Check sheet for the modelled part. Datum: model origin and axes. Units: mm. Face numbers are marked on the shaded views. Give positions to 0.01 mm unless a question says otherwise; leave off trailing zeros. Write each loop counter-clockwise with the first axis right and the second up, starting at its lowest first coordinate (ties: lowest second). Pieces come first, ordered by that corner, then holes. Notation, with made-up numbers: (51.5, 33) -> (62.5, 33) arc R21 ccw to (62.5, 39) -> close; hole circle Ø6 at (34.25, 73). An arc over 180 degrees is marked (long way). Use a Markdown table: item, result. Add a question column.
1. Cross-section at B-B (x = 0). Enter the section's corners in (y, z).
2. Cross-section at A-A (y = 0). Enter the section's corners in (x, z).
3. Scan lines: probe 1 along Y at (x, z) = (0, 12.5); probe 2 along Z at (x, y) = (7, 16.5); probe 3 along X at (y, z) = (-14, 8.25). Record each from-to range of solid material in increasing order. Write a range as [from, to].
4. Release check for a two-part mould opening along X. For the marked faces 1, 2 and 3 record: released by +X, released by -X, zero draft, split by the parting line, or undercut.
5. Cross-section at C-C (z = 9). Enter the section's corners in (x, y), then the cut area to 3 significant figures.
6. Gauge pin test, flat ends, axial feed: P1, Ø1.1, axis at x = -28, z = 15, coming from the -Y side; P2, Ø10, axis at x = -13.5, z = 7, coming from the +Y side; P3, Ø1.6, axis at x = 19.5, z = 19, coming from the -Y side; P4, Ø6, axis at x = -10.5, z = 3, coming from the -Y side. Record the tip position at first contact, or that the pin passes through.
from build123d import *

# Parameters (mm, degrees)
F0_R      = 29
F4_DEPTH  = 20
F5_SIZE   = 1
F1_R      = 28
F6_DEPTH  = 18
F2_W      = 5
F2_H      = 14
F7_DEPTH  = 20.1
F3_W      = 10.5
F3_H      = 2.55
F8_DEPTH  = 42.4
F9_W      = 46.34465
F9_H      = 65.188974
F10_DEPTH = 7
F11_W     = 30
F11_H     = 4
F12_DEPTH = 45


with BuildPart() as f4:
    # F0 (on Top) → F4 (new body)
    with BuildSketch(Plane.XY):
        Circle(F0_R)
    extrude(amount=F4_DEPTH)

    # F5
    f5_edges = [f4.edges().sort_by_distance(p)[0] for p in [
        (-29, 0, 20),
    ]]
    chamfer(f5_edges, length=F5_SIZE)

    # F1 (on Top) → F6 (cut)
    with BuildSketch(Plane.XY):
        Circle(F1_R)
    extrude(amount=F6_DEPTH, mode=Mode.SUBTRACT)

    # F2 (on face) → F7 (cut)
    with BuildSketch(Plane.XY):
        with Locations((18.5, 8.5)):
            Rectangle(F2_W, F2_H)
        with Locations((18.5, -8.5)):
            Rectangle(F2_W, F2_H)
    extrude(amount=F7_DEPTH, mode=Mode.SUBTRACT)

    # F3 (on Right) → F8 (cut)
    with BuildSketch(Plane.YZ):
        with Locations((-11.250031, 14.775)):
            Rectangle(F3_W, F3_H)
    extrude(amount=-F8_DEPTH, mode=Mode.SUBTRACT)

    # F9 (on Top) → F10 (cut)
    with BuildSketch(Plane.XY):
        Rectangle(F9_W, F9_H)
    extrude(amount=F10_DEPTH, mode=Mode.SUBTRACT)

    # F11 (on Right) → F12 (cut, symmetric)
    with BuildSketch(Plane.YZ):
        with Locations((0, 4)):
            Rectangle(F11_W, F11_H)
    extrude(amount=F12_DEPTH, both=True, mode=Mode.SUBTRACT)


solid = f4.part
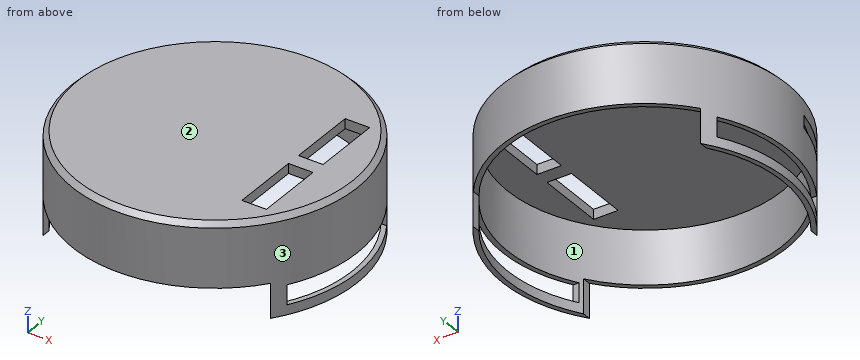
Worked answers:
| question | item | result |
|---|---|---|
| 1 | outline | (-29, 7) -> (-28, 7) -> (-28, 18) -> (28, 18) -> (28, 7) -> (29, 7) -> (29, 19) -> (28, 20) -> (-28, 20) -> (-29, 19) -> close |
| 2 | outline | (-29, 0) -> (-28, 0) -> (-28, 2) -> (-29, 2) -> close; (-29, 6) -> (-28, 6) -> (-28, 18) -> (28, 18) -> (28, 6) -> (29, 6) -> (29, 19) -> (28, 20) -> (-28, 20) -> (-29, 19) -> close; (28, 0) -> (29, 0) -> (29, 2) -> (28, 2) -> close |
| 3 | probe 1 | y = [-29, -28], [28, 29] |
| 3 | probe 2 | z = [18, 20] |
| 3 | probe 3 | x = [-25.4, -24.25], [24.25, 25.4] |
| 4 | face 1 | undercut |
| 4 | face 2 | zero draft |
| 4 | face 3 | split by the parting line |
| 5 | outline | circle Ø58 at (0, 0); hole circle Ø56 at (0, 0) |
| 5 | area | 179 mm² |
| 6 | P1 | stops at y = -6 |
| 6 | P2 | stops at y = 27.73 |
| 6 | P3 | stops at y = -22.17 |
| 6 | P4 | passes through |
